from build123d import *

# Parameters (mm, degrees)
SKETCH2_W           = 250
SKETCH2_H           = 200
BOSS_EXTRUDE2_DEPTH = 3
SKETCH3_R           = 1.75
SKETCH3_R_2         = 3.3
SKETCH3_R_3         = 1.7
SKETCH3_R_4         = 1.2
SKETCH3_R_5         = 1.6
SKETCH3_R_6         = 1.1
SKETCH3_W           = 13.2
SKETCH3_H           = 19.2
CUT_EXTRUDE1_DEPTH  = 3


with BuildPart() as part:
    # Sketch2 → Boss-Extrude2 (new body)
    with BuildSketch(Plane(origin=(0, 0, 0), x_dir=(1, 0, 0), z_dir=(0, 1, 0))):
        Rectangle(SKETCH2_W, SKETCH2_H)
    extrude(amount=BOSS_EXTRUDE2_DEPTH)

    # Sketch3 → Cut-Extrude1 (cut)
    with BuildSketch(Plane(origin=(0, 3, 0), x_dir=(1, 0, 0), z_dir=(0, 1, 0))):
        with Locations(Location((-105, 85, 0), (0, 0, 270))):
            Circle(SKETCH3_R)
        with Locations(Location((-15, 85, 0), (0, 0, 270))):
            Circle(SKETCH3_R)
        with Locations(Location((-117, 92, 0), (0, 0, 270))):
            Circle(SKETCH3_R_2)
        with Locations(Location((-117, -92, 0), (0, 0, 90))):
            Circle(SKETCH3_R_2)
        with Locations(Location((117, 92, 0), (0, 0, 90))):
            Circle(SKETCH3_R_2)
        with Locations(Location((117, -92, 0), (0, 0, 270))):
            Circle(SKETCH3_R_2)
        with Locations(Location((-75, 50, 0), (0, 0, 270))):
            Circle(SKETCH3_R_3)
        with Locations(Location((-17, 50, 0), (0, 0, 270))):
            Circle(SKETCH3_R_3)
        with Locations(Location((-75, 19, 0), (0, 0, 270))):
            Circle(SKETCH3_R_3)
        with Locations(Location((-17, 19, 0), (0, 0, 270))):
            Circle(SKETCH3_R_3)
        with Locations(Location((95, 60, 0), (0, 0, 270))):
            Circle(SKETCH3_R_3)
        with Locations(Location((95, 23.07, 0), (0, 0, 270))):
            Circle(SKETCH3_R_3)
        with Locations(Location((96, -40, 0), (0, 0, 270))):
            Circle(SKETCH3_R_4)
        with Locations(Location((115, -40, 0), (0, 0, 270))):
            Circle(SKETCH3_R_4)
        with Locations(Location((115, -78.4, 0), (0, 0, 270))):
            Circle(SKETCH3_R_4)
        with Locations(Location((96, -78.4, 0), (0, 0, 270))):
            Circle(SKETCH3_R_4)
        with Locations(Location((-39.35, -10, 0), (0, 0, 270))):
            Circle(SKETCH3_R_5)
        with Locations(Location((39.35, -10, 0), (0, 0, 270))):
            Circle(SKETCH3_R_5)
        with Locations(Location((-39.35, -90, 0), (0, 0, 270))):
            Circle(SKETCH3_R_5)
        with Locations(Location((39.35, -90, 0), (0, 0, 270))):
            Circle(SKETCH3_R_5)
        with Locations(Location((-36.85, -27.75, 0), (0, 0, 270))):
            Circle(SKETCH3_R_6)
        with Locations(Location((36.85, -27.75, 0), (0, 0, 270))):
            Circle(SKETCH3_R_6)
        with Locations(Location((36.85, -72.25, 0), (0, 0, 270))):
            Circle(SKETCH3_R_6)
        with Locations(Location((-36.85, -72.25, 0), (0, 0, 270))):
            Circle(SKETCH3_R_6)
        with Locations((-108.4, 50.4)):
            Rectangle(SKETCH3_W, SKETCH3_H)
    extrude(amount=-CUT_EXTRUDE1_DEPTH, mode=Mode.SUBTRACT)


solid = part.part
Verification items for the finished model (mm, model axes). Give positions to 0.01 mm unless a question says otherwise; leave off trailing zeros. Loops run counter-clockwise (first coordinate to the right, second up) from the corner with the lowest first, then second, coordinate; pieces in that order, holes last.
1) Sectioned sample at A-A, the plane z = -92. Enter the section's corners in (x, y), then the cut area to 3 significant figures.
2) Draft check along Z on faces 1 (the flat face through (-2, 3, -1)), 2 (the cylindrical face through (119.008, 1.521, -89.381)). Enter one of: pulls with the +Z half, pulls with the -Z half, needs draft (parallel to the pull), parting line crosses it, or undercut.
3) Depth check by flat-ended pin: pin 1 Ø3 at (x, z) = (96, 40) entering from +Y; pin 2 Ø1.3 at (x, z) = (-36.85, 72.25) entering from +Y. Enter the tip coordinate at first touch or a pass-through.
4) Thickness scan on line 1 along Z through (x, y) = (39, 0.9); line 2 along Z through (x, y) = (-75, 1.9); line 3 along X through (y, z) = (1.3, 40). Record the ranges inside material, lowest first.
Answers:
1. outline: (-125, 0) - (-120.3, 0) - (-120.3, 3) - (-125, 3) - close; (-113.7, 0) - (113.7, 0) - (113.7, 3) - (-113.7, 3) - close; (120.3, 0) - (125, 0) - (125, 3) - (120.3, 3) - close
1. area: 710 mm2
2. face 1: needs draft
2. face 2: undercut
3. pin 1: stops at y = 3
3. pin 2: passes through
4. line 1: z = -100 to 8.44, 11.56 to 88.44, 91.56 to 100
4. line 2: z = -100 to -51.7, -48.3 to -20.7, -17.3 to 100
4. line 3: x = -125 to 94.8, 97.2 to 113.8, 116.2 to 125
